```python
from build123d import *

# Parameters (mm, degrees)
BOSS_EXTRUDE1_DEPTH = 3
SKETCH2_R           = 4.5
BOSS_EXTRUDE2_DEPTH = 6
CUT_EXTRUDE1_REACH  = 35.068
SKETCH3_R           = 2
SKETCH4_R           = 2.5
CUT_EXTRUDE2_DEPTH  = 0.5
BOSS_EXTRUDE4_DEPTH = 9
CHAMFER1_SIZE       = 0.3
FILLET1_R           = 0.2


with BuildPart() as part:
    # Sketch1 → Boss-Extrude1 (new body)
    with BuildSketch(Plane(origin=(0, 0, 0), x_dir=(1, 0, 0), z_dir=(0, 1, 0))):
        with BuildLine():
            Line((-27, 4.5), (27, 4.5))
            ThreePointArc((27, 4.5), (31.5, 0), (27, -4.5))
            Line((27, -4.5), (-27, -4.5))
            ThreePointArc((-27, -4.5), (-31.5, 0), (-27, 4.5))
        make_face()
    extrude(amount=-BOSS_EXTRUDE1_DEPTH)

    # Sketch2 → Boss-Extrude2 (add)
    with BuildSketch(Plane(origin=(0, 0, 0), x_dir=(1, 0, 0), z_dir=(0, 1, 0))):
        with Locations(Location((-27, 0, 0), (0, 0, 270))):
            Circle(SKETCH2_R)
        with Locations(Location((27, 0, 0), (0, 0, 270))):
            Circle(SKETCH2_R)
    extrude(amount=BOSS_EXTRUDE2_DEPTH)

    # Sketch3 → Cut-Extrude1 (cut, up to next)
    with BuildSketch(Plane(origin=(0, 6, 0), x_dir=(1, 0, 0), z_dir=(0, 1, 0)), mode=Mode.PRIVATE) as cut_extrude1_sk1:
        with Locations(Location((-27, 0, 0), (0, 0, 270))):
            Circle(SKETCH3_R)
    cut_extrude1_tool1 = extrude(cut_extrude1_sk1.sketch, amount=-CUT_EXTRUDE1_REACH, mode=Mode.PRIVATE) & part.part
    # Sketch3 → Cut-Extrude1 (cut, up to next)
    with BuildSketch(Plane(origin=(0, 6, 0), x_dir=(1, 0, 0), z_dir=(0, 1, 0)), mode=Mode.PRIVATE) as cut_extrude1_sk2:
        with Locations(Location((27, 0, 0), (0, 0, 270))):
            Circle(SKETCH3_R)
    cut_extrude1_tool2 = extrude(cut_extrude1_sk2.sketch, amount=-CUT_EXTRUDE1_REACH, mode=Mode.PRIVATE) & part.part
    add(cut_extrude1_tool1.solids().sort_by_distance((-27, 6, 0))[0], mode=Mode.SUBTRACT)
    add(cut_extrude1_tool2.solids().sort_by_distance((27, 6, 0))[0], mode=Mode.SUBTRACT)

    # Sketch4 → Cut-Extrude2 (cut)
    with BuildSketch(Plane(origin=(0, 6, 0), x_dir=(1, 0, 0), z_dir=(0, 1, 0))):
        with Locations(Location((-27, 0, 0), (0, 0, 270))):
            Circle(SKETCH4_R)
        with Locations(Location((27, 0, 0), (0, 0, 90))):
            Circle(SKETCH4_R)
    cut_extrude2 = extrude(amount=-CUT_EXTRUDE2_DEPTH, mode=Mode.SUBTRACT)

    # Mirror1: Cut-Extrude2 across plane
    add(cut_extrude2.mirror(Plane(origin=(0, 1.5, 0), x_dir=(0, 0, 1), z_dir=(0, -1, 0))), mode=Mode.SUBTRACT)

    # Sketch21 → Boss-Extrude4 (add)
    with BuildSketch(Plane.XY.offset(4.5)):
        Polygon((-20, 0), (-18, 0), (-18.5, 2.5), (-19.5, 2.5), align=None)
        Polygon((-16.831620529, 0), (-16.331620529, 2.5), (-15.331620529, 2.5), (-14.831620529, 0), align=None)
        Polygon((-13.663241058, 0), (-13.163241058, 2.5), (-12.163241058, 2.5), (-11.663241058, 0), align=None)
        Polygon((-10.494861587, 0), (-9.994861587, 2.5), (-8.994861587, 2.5), (-8.494861587, 0), align=None)
        Polygon((-7.326482116, 0), (-6.826482116, 2.5), (-5.826482116, 2.5), (-5.326482116, 0), align=None)
        Polygon((-4.158102645, 0), (-3.658102645, 2.5), (-2.658102645, 2.5), (-2.158102645, 0), align=None)
        Polygon((-0.989723174, 0), (-0.489723174, 2.5), (0.510276826, 2.5), (1.010276826, 0), align=None)
        Polygon((2.178656297, 0), (2.678656297, 2.5), (3.678656297, 2.5), (4.178656297, 0), align=None)
        Polygon((5.347035768, 0), (5.847035768, 2.5), (6.847035768, 2.5), (7.347035768, 0), align=None)
        Polygon((8.515415239, 0), (9.015415239, 2.5), (10.015415239, 2.5), (10.515415239, 0), align=None)
        Polygon((11.68379471, 0), (12.18379471, 2.5), (13.18379471, 2.5), (13.68379471, 0), align=None)
        Polygon((14.852174181, 0), (15.352174181, 2.5), (16.352174181, 2.5), (16.852174181, 0), align=None)
        Polygon((18.020553652, 0), (18.520553652, 2.5), (19.520553652, 2.5), (20.020553652, 0), align=None)
    extrude(amount=-BOSS_EXTRUDE4_DEPTH)

    # Chamfer1
    chamfer1_edges = [part.edges().sort_by_distance(p)[0] for p in [
        (-6.326482116, 2.5, 4.5),
        (-6.326482116, 2.5, -4.5),
        (-3.158102645, 2.5, 4.5),
        (-3.158102645, 2.5, -4.5),
        (0.010276826, 2.5, 4.5),
        (0.010276826, 2.5, -4.5),
        (3.178656297, 2.5, 4.5),
        (3.178656297, 2.5, -4.5),
        (6.347035768, 2.5, 4.5),
        (6.347035768, 2.5, -4.5),
        (9.515415239, 2.5, 4.5),
        (9.515415239, 2.5, -4.5),
        (12.68379471, 2.5, 4.5),
        (12.68379471, 2.5, -4.5),
        (15.852174181, 2.5, 4.5),
        (15.852174181, 2.5, -4.5),
        (19.020553652, 2.5, 4.5),
        (19.020553652, 2.5, -4.5),
        (-19, 2.5, 4.5),
        (-19, 2.5, -4.5),
        (-15.831620529, 2.5, 4.5),
        (-15.831620529, 2.5, -4.5),
        (-12.663241058, 2.5, 4.5),
        (-12.663241058, 2.5, -4.5),
        (-9.494861587, 2.5, 4.5),
        (-9.494861587, 2.5, -4.5),
    ]]
    chamfer(chamfer1_edges, length=CHAMFER1_SIZE)

    # Fillet1
    fillet1_edges = [part.edges().sort_by_distance(p)[0] for p in [
        (-27, 6, -4.5),
        (27, 6, -4.5),
    ]]
    fillet(fillet1_edges, radius=FILLET1_R)


solid = part.part
```
Check sheet for the modelled part. Datum: model origin and axes. Units: mm. A direction names the side the tool comes from. Round coordinates to 2 decimals unless told otherwise and drop trailing zeros. Order: outer loops, then holes, each group sorted by start corner. A loop starts at its lowest first (then second) coordinate and runs counter-clockwise, first axis right, second up.
1) Tool access check on faces 1 (the flat face through (25, 5.5, 1)), 2 (the flat face through (10.26, 1.27, 0.06)), 3 (the flat face through (-25, -2.5, -1)), 4 (the cylindrical face through (25, 2, 0)). Record the directions out of +Z, -Z, +X, -X, +Y, -Y that give a thin tool (end or side, any length) a straight path to the whole face; none if there is none.
2) Section check A-A (z = 0). Give the number of separate pieces and of enclosed holes in the cut face, and give its area (3 significant figures).
3) Section check B-B (y = 4.25). Record the boundary of the cut face in (x, z).
4) Scan lines: line 1 (Z direction, x = 27, y = 5.75); line 2 (X direction, y = -2.7, z = 0); line 3 (X direction, y = 4.75, z = -1.25). Record each from-to range of solid material in increasing order.
5) Section check D-D (x = 21.5). Record the boundary of the cut face in (y, z), and give its area (3 significant figures).
6) Go/stop test with flat-tipped pins: pin 1 Ø1.5 at (x, z) = (-7.5, -3) entering from +Y; pin 2 Ø0.6 at (x, z) = (-17.5, 0) entering from +Y; pin 3 Ø5 at (y, z) = (5, 0.5) entering from -X; pin 4 Ø2 at (y, z) = (2, 3) entering from -X. Record where each tip stops, or that it passes through.
Result:
1. face 1: +Y
1. face 2: +Z, -Z, +Y
1. face 3: -Y
1. face 4: +Y, -Y
2. separate pieces: 3
2. enclosed holes: 0
2. area: 272 mm2
3. outline: circle Ø9 at (-27, 0); circle Ø9 at (27, 0); hole circle Ø4 at (-27, 0); hole circle Ø4 at (27, 0)
4. line 1: z = -4.5 to -2.5, 2.5 to 4.5
4. line 2: x = -31.5 to -29.5, -24.5 to 24.5, 29.5 to 31.5
4. line 3: x = -31.32 to -28.56, -25.44 to -22.68, 22.68 to 25.44, 28.56 to 31.32
5. outline: (-3, -4.5) - (0, -4.5) - (0, 4.5) - (-3, 4.5) - close
5. area: 27.0 mm2
6. pin 1: stops at y = 2.5
6. pin 2: stops at y = 0
6. pin 3: stops at x = -31.5
6. pin 4: stops at x = -31.03
